Read the model definition and answer for the solid it produces. Units are mm, in the model's axes. A direction names the side the tool comes from. Coordinates: 2 decimals unless noted, no trailing zeros. Loops run counter-clockwise (first coordinate to the right, second up) from the corner with the lowest first, then second, coordinate; pieces in that order, holes last. Notation, with made-up numbers: M 50.25,-20 L 55.25,-20 A30 ccw 55.25,11 Z; hole C -2.5,-8.75 d2. An arc over 180 degrees is marked long. Put each result on its own line as item: value.
from build123d import *

# Parameters (mm, degrees)
BOSS_EXTRUDE1_DEPTH              = 6.35
CUT_EXTRUDE1_DEPTH               = 221.472033966
F_27_64_0_42188_DIAMETER_HOLE1_D = 10.715752
FILLET1_R                        = 2.54
F_1_2_CLEARANCE_HOLE1_D          = 13.49248


with BuildPart() as part:
    # Sketch1 → Boss-Extrude1 (new body)
    with BuildSketch(Plane.XY):
        with BuildLine():
            Line((-179.07, -25.4), (-179.07, 128.45828257))
            Line((-179.07, 128.45828257), (179.07, 128.45828257))
            Line((179.07, 128.45828257), (179.07, -25.4))
            Line((179.07, -25.4), (153.67, -25.4))
            Line((153.67, -25.4), (153.67, -1.27))
            ThreePointArc((153.67, -1.27), (127, 25.4), (100.33, -1.27))
            Line((100.33, -1.27), (100.33, -25.4))
            Line((100.33, -25.4), (-100.33, -25.4))
            Line((-100.33, -25.4), (-100.33, -1.27))
            ThreePointArc((-100.33, -1.27), (-127, 25.4), (-153.67, -1.27))
            Line((-153.67, -1.27), (-153.67, -25.4))
            Line((-153.67, -25.4), (-179.07, -25.4))
        make_face()
    extrude(amount=BOSS_EXTRUDE1_DEPTH)

    # Sketch7 → Cut-Extrude1 (cut, through all)
    with BuildSketch(Plane(origin=(0, 0, 0), x_dir=(-1, 0, 0), z_dir=(0, 0, -1))):
        with BuildLine():
            Line((-151.892, 128.45828257), (-151.892, 8.304823027))
            ThreePointArc((-151.892, 8.304823027), (-153.22173278, 3.599253536), (-153.67, -1.27))
            Line((-153.67, -1.27), (-153.67, -25.4))
            Line((-153.67, -25.4), (-179.07, -25.4))
            Line((-179.07, -25.4), (-179.07, 128.45828257))
            Line((-179.07, 128.45828257), (-151.892, 128.45828257))
        make_face()
        with BuildLine():
            Line((153.67, -25.4), (153.67, -1.27))
            ThreePointArc((153.67, -1.27), (153.22173278, 3.599253536), (151.892, 8.304823027))
            Line((151.892, 8.304823027), (151.892, 128.45828257))
            Line((151.892, 128.45828257), (179.07, 128.45828257))
            Line((179.07, 128.45828257), (179.07, -25.4))
            Line((179.07, -25.4), (153.67, -25.4))
        make_face()
    extrude(amount=-CUT_EXTRUDE1_DEPTH, mode=Mode.SUBTRACT)

    # 27/64 (0.42188) Diameter Hole1 (through all)
    with Locations(Plane.XY.offset(6.35)):
        with Locations((-97.79, 34.29), (-97.79, 112.58328257), (97.79, 34.29), (97.79, 112.58328257)):
            Hole(F_27_64_0_42188_DIAMETER_HOLE1_D / 2)

    # Fillet1
    fillet1_edges = [part.edges().sort_by_distance(p)[0] for p in [
        (100.33, -25.4, 3.175),
        (-100.33, -25.4, 3.175),
        (151.892, 128.45828257, 3.175),
        (151.892, 8.304823027, 3.175),
        (-151.892, 8.304823027, 3.175),
        (-151.892, 128.45828257, 3.175),
    ]]
    fillet(fillet1_edges, radius=FILLET1_R)

    # 1/2 Clearance Hole1 (through all)
    with Locations(Plane.XY.offset(6.35)):
        with Locations((57.15, 69.85), (-57.15, 69.85)):
            Hole(F_1_2_CLEARANCE_HOLE1_D / 2)


solid = part.part
1) Given pin 1 Ø3 at (y, z) = (-10.5, 4.5) entering from +X; pin 2 Ø3 at (y, z) = (-7.5, 4) entering from -X, each flat-ended and moving along its own axis, determine where each tip first touches the part or whether it passes through.
Answer list:
pin 1: stops at x = 100.33
pin 2: stops at x = -100.33
2) Find section C-C, the plane z = 2. Write down the section's boundary in (x, y).
Answer list:
outline: M -151.89,17.53 A2.54 ccw -147.41,15.9 A26.67 cw -100.33,-1.27 L -100.33,-22.86 A2.54 ccw -97.79,-25.4 L 97.79,-25.4 A2.54 ccw 100.33,-22.86 L 100.33,-1.27 A26.67 cw 147.41,15.9 A2.54 ccw 151.89,17.53 L 151.89,125.92 A2.54 ccw 149.35,128.46 L -149.35,128.46 A2.54 ccw -151.89,125.92 Z; hole C -97.79,34.29 d10.72; hole C -97.79,112.58 d10.72; hole C -57.15,69.85 d13.49; hole C 57.15,69.85 d13.49; hole C 97.79,34.29 d10.72; hole C 97.79,112.58 d10.72
3) Determine the mould class of faces 3 (the flat face through (-100.33, -12, 3)), 4 (the cylindrical face through (92.84, 110.53, 3.13)), 5 (the cylindrical face through (-96.629, 107.353, 3.131)), 6 (the flat face through (151.892, 72, 3)) for opening direction X: released by +X, released by -X, zero draft, split by the parting line, or undercut.
Answer list:
face 3: released by -X
face 4: undercut
face 5: undercut
face 6: released by +X
4) Find section D-D, the plane y = -6.5. Write down the section's boundary in (x, z).
Answer list:
outline: M -100.33,0 L 100.33,0 L 100.33,6.35 L -100.33,6.35 Z
5) Straight lines are drawn through the part: line 1 (Y direction, x = 97.79, z = 2.75); line 2 (Y direction, x = -57.15, z = 4.75); line 3 (Y direction, x = -128, z = 5). For each, find the intervals that lie inside material, in ascending order. Write a range as [from, to].
Answer list:
line 1: y = [-25.4, 28.93], [39.65, 107.23], [117.94, 128.46]
line 2: y = [-25.4, 63.1], [76.6, 128.46]
line 3: y = [25.38, 128.46]
6) Find section B-B, the plane x = -57.15. Write down the section's boundary in (y, z).
Answer list:
outline: M -25.4,0 L 63.1,0 L 63.1,6.35 L -25.4,6.35 Z; M 76.6,0 L 128.46,0 L 128.46,6.35 L 76.6,6.35 Z
7) Find section A-A, the plane y = 34.29. Write down the section's boundary in (x, z).
Answer list:
outline: M -151.89,0 L -103.15,0 L -103.15,6.35 L -151.89,6.35 Z; M -92.43,0 L 92.43,0 L 92.43,6.35 L -92.43,6.35 Z; M 103.15,0 L 151.89,0 L 151.89,6.35 L 103.15,6.35 Z
8) Which of the six approach directions +Z, -Z, +X, -X, +Y, -Y give full straight-line access (tool end or side, diameter ignored) to faces 1 (the flat face through (100.33, -12, 3)), 2 (the flat face through (1, -25.4, 3))?
Answer list:
face 1: +Z, -Z, +X, -Y
face 2: +Z, -Z, +X, -X, -Y
